Design review of the part built by this model. Coordinates are the model's own, in mm. Coordinates: 2 decimals unless noted, no trailing zeros. Write each loop counter-clockwise with the first axis right and the second up, starting at its lowest first coordinate (ties: lowest second). Pieces come first, ordered by that corner, then holes. Notation, with made-up numbers: (77, 10.5) - (136, 10.5) arc R19 cw to (136, 45.5) - close; hole circle Ø10 at (81.25, 49.25). An arc over 180 degrees is marked (long way). Use a Markdown table: item, result.
from build123d import *

# Parameters (mm, degrees)
SKETCH1_R           = 30.5
BOSS_EXTRUDE1_DEPTH = 2
SKETCH2_R           = 2
CUT_EXTRUDE1_DEPTH  = 44.179856415
SKETCH4_R           = 0.5
CUT_EXTRUDE2_DEPTH  = 44.179856415
CUT_EXTRUDE3_DEPTH  = 0.5


with BuildPart() as part:
    # Sketch1 → Boss-Extrude1 (new body)
    with BuildSketch(Plane(origin=(0, 0, 0), x_dir=(1, 0, 0), z_dir=(0, 1, 0))):
        with Locations(Location((0, 0, 0), (0, 0, 270))):
            Circle(SKETCH1_R)
    extrude(amount=BOSS_EXTRUDE1_DEPTH)

    # Sketch2 → Cut-Extrude1 (cut, through all)
    with BuildSketch(Plane(origin=(0, 2, 0), x_dir=(1, 0, 0), z_dir=(0, 1, 0))):
        with Locations(Location((0, 0, 0), (0, 0, 270))):
            Circle(SKETCH2_R)
    extrude(amount=-CUT_EXTRUDE1_DEPTH, mode=Mode.SUBTRACT)

    # Sketch4 → Cut-Extrude2 (cut, through all)
    with BuildSketch(Plane(origin=(0, 2, 0), x_dir=(1, 0, 0), z_dir=(0, 1, 0))):
        with Locations(Location((0, 15, 0), (0, 0, 270))):
            Circle(SKETCH4_R)
        with Locations(Location((0, -15, 0), (0, 0, 90))):
            Circle(SKETCH4_R)
    extrude(amount=-CUT_EXTRUDE2_DEPTH, mode=Mode.SUBTRACT)

    # Sketch5 → Cut-Extrude3 (cut)
    with BuildSketch(Plane.XZ):
        with BuildLine():
            Line((0.599999999, 26), (0.599999999, 15))
            ThreePointArc((0.599999999, 15), (0, 14.400000002), (-0.599999999, 15))
            Line((-0.599999999, 15), (-0.599999999, 26))
            ThreePointArc((-0.599999999, 26), (0, 26.599999999), (0.599999999, 26))
        make_face()
        with BuildLine():
            Line((0.599999999, -26), (0.599999999, -15.000000001))
            ThreePointArc((0.599999999, -15.000000001), (0, -14.400000003), (-0.599999999, -15.000000001))
            Line((-0.599999999, -15.000000001), (-0.599999999, -26))
            ThreePointArc((-0.599999999, -26), (0, -26.6), (0.599999999, -26))
        make_face()
    extrude(amount=-CUT_EXTRUDE3_DEPTH, mode=Mode.SUBTRACT)


solid = part.part
(1) Take a section at D-D on x = 12. Write out the cut boundary in (y, z).
Determined:
| item | result |
|---|---|
| outline | (0, -28.04) - (2, -28.04) - (2, 28.04) - (0, 28.04) - close |
(2) Take a section at B-B on y = 1.2. Write out the cut boundary in (x, z), and give its area (3 significant figures).
Determined:
| item | result |
|---|---|
| outline | circle Ø61 at (0, 0); hole circle Ø4 at (0, 0); hole circle Ø1 at (0, -15); hole circle Ø1 at (0, 15) |
| area | 2,910 mm2 |
(3) Draft analysis for pull direction X (two halves, no side actions). For faces 1 (the flat face through (-6, 0, 0)), 2 (the cylindrical face through (-2, 1, 0)), 3 (the cylindrical face through (-29.775, 0.986, -6.612)), state which applies: +X half, -X half, draft (parallel to the pull), parting line (faces both ways), or undercut.
Determined:
| item | result |
|---|---|
| face 1 | draft |
| face 2 | undercut |
| face 3 | parting line |
(4) For L1, parallel to X at y = 1.65, z = -15; L2, parallel to Z at x = -13.5, y = 0.35; L3, parallel to X at y = 1.75, z = 16, list the stretches that pass through material, from the lowest coordinate up. Write a range as from..to.
Determined:
| item | result |
|---|---|
| L1 | -26.56..-0.5, 0.5..26.56 |
| L2 | -27.35..27.35 |
| L3 | -25.97..25.97 |
(5) Take a section at C-C on z = 19. Write out the cut boundary in (x, y), and give its area (3 significant figures).
Determined:
| item | result |
|---|---|
| outline | (-23.86, 0) - (-0.6, 0) - (-0.6, 0.5) - (0.6, 0.5) - (0.6, 0) - (23.86, 0) - (23.86, 2) - (-23.86, 2) - close |
| area | 94.8 mm2 |
(6) For pin 1 (1 mm diameter, centred on y = 0.5, z = -1, fed in from +X), flat-tipped, find the tip position at first contact; note if it passes through.
Determined:
| item | result |
|---|---|
| pin 1 | x = 30.5 |
(7) Take a section at A-A on z = 0. Write out the cut boundary in (x, y).
Determined:
| item | result |
|---|---|
| outline | (-30.5, 0) - (-2, 0) - (-2, 2) - (-30.5, 2) - close; (2, 0) - (30.5, 0) - (30.5, 2) - (2, 2) - close |
